```python
from build123d import *

# Parameters (mm, degrees)
F0_W     = 1500
F0_H     = 1000
F1_DEPTH = 1500
F2_W     = 300
F2_H     = 80
F3_DEPTH = 1000
F4_W     = 290.798738
F4_H     = 1259.663105
F4_W_2   = 753.015757
F5_DEPTH = 25
F6_W     = 1170.94978
F6_H     = 737.592996
F7_DEPTH = 25
F8_W     = 501.033828
F8_H     = 1276.894093
F9_DEPTH = 25


with BuildPart() as f1:
    # F0 (on Front) → F1 (new body)
    with BuildSketch(Plane.XZ):
        with Locations((750, 500)):
            Rectangle(F0_W, F0_H)
    extrude(amount=F1_DEPTH)

    # F2 (on face) → F3 (cut)
    with BuildSketch(Plane.XY.offset(1000)):
        with Locations((250, -1460)):
            Rectangle(F2_W, F2_H)
        with Locations((1250, -1460)):
            Rectangle(F2_W, F2_H)
    extrude(amount=-F3_DEPTH, mode=Mode.SUBTRACT)

    # F4 (on face) → F5 (cut)
    with BuildSketch(Plane.XY.offset(1000)):
        with Locations((286.252491, -629.831552)):
            Rectangle(F4_W, F4_H)
        with Locations((988.761067, -629.831552)):
            Rectangle(F4_W_2, F4_H)
    extrude(amount=-F5_DEPTH, mode=Mode.SUBTRACT)

    # F6 (on face) → F7 (cut)
    with BuildSketch(Plane(origin=(0, 0, 0), x_dir=(0, -1, 0), z_dir=(-1, 0, 0))):
        with Locations((685.361821, 483.926624)):
            Rectangle(F6_W, F6_H)
    extrude(amount=-F7_DEPTH, mode=Mode.SUBTRACT)

    # F8 (on face) → F9 (cut)
    with BuildSketch(Plane(origin=(0, 0, 0), x_dir=(1, 0, 0), z_dir=(0, 0, -1))):
        with Locations((446.271874, 638.447046)):
            Rectangle(F8_W, F8_H)
    extrude(amount=-F9_DEPTH, mode=Mode.SUBTRACT)


solid = f1.part
```
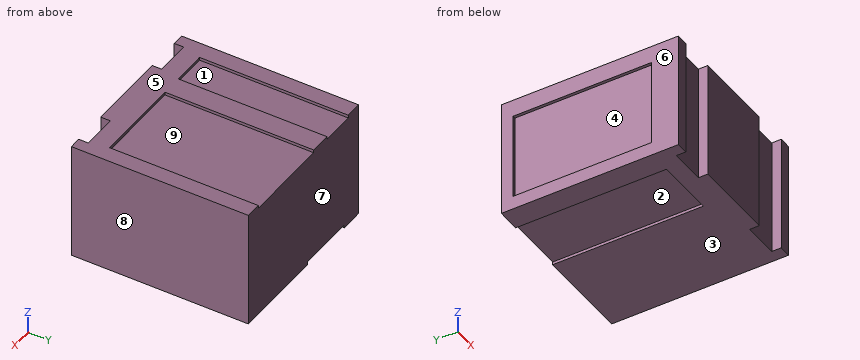
Design review of the part built by this model. Coordinates are the model's own, in mm. Face numbers are marked on the shaded views. A direction names the side the tool comes from. Round coordinates to 2 decimals unless told otherwise and drop trailing zeros. Write each loop counter-clockwise with the first axis right and the second up, starting at its lowest first coordinate (ties: lowest second). Pieces come first, ordered by that corner, then holes.
Item 1: We need section B-B on x = 348. Write out the cut boundary in (y, z).
Item 2: Clearance check with flat-ended pins moving along their axes: pin 1 Ø10 at (x, y) = (469.5, -856) entering from -Z; pin 2 Ø5 at (y, z) = (-514.5, 172) entering from -X; pin 3 Ø1.5 at (x, z) = (1220, 791.5) entering from -Y. State where each tip first meets the part, or that it passes through.
Item 3: We need section D-D on z = 932. Write out the cut boundary in (x, y).
Item 4: We need section C-C on y = -757. Write out the cut boundary in (x, z).
Item 5: The part is to be moulded in two halves that separate along X. For the marked faces 6, 7, 8 and 9, say which applies: +X half, -X half, draft (parallel to the pull), parting line (faces both ways), or undercut.
Item 6: For probe 1 along X at (y, z) = (-575, 244.5); probe 2 along Z at (x, y) = (1089, -923); probe 3 along Y at (x, z) = (219, 958.5), list the stretches that pass through material, from the lowest coordinate up.
Item 7: We need section A-A on z = 773. Write out the cut boundary in (x, y).
Item 8: For the marked faces 1, 2, 3, 4 and 5, list the 3-axis set-ups (+Z, -Z, +X, -X, +Y, -Y) from which the entire face can be reached by the end or side of a thin tool; tool diameter is ignored.
Returned:
1. outline: (-1420, 0) - (-1276.89, 0) - (-1276.89, 25) - (0, 25) - (0, 975) - (-1259.66, 975) - (-1259.66, 1000) - (-1420, 1000) - close
2. pin 1: stops at z = 25
2. pin 2: stops at x = 25
2. pin 3: stops at y = -1420
3. outline: (0, -1500) - (100, -1500) - (100, -1420) - (400, -1420) - (400, -1500) - (1100, -1500) - (1100, -1420) - (1400, -1420) - (1400, -1500) - (1500, -1500) - (1500, 0) - (0, 0) - close
4. outline: (0, 0) - (195.75, 0) - (195.75, 25) - (696.79, 25) - (696.79, 0) - (1500, 0) - (1500, 1000) - (1365.27, 1000) - (1365.27, 975) - (612.25, 975) - (612.25, 1000) - (431.65, 1000) - (431.65, 975) - (140.85, 975) - (140.85, 1000) - (0, 1000) - (0, 852.72) - (25, 852.72) - (25, 115.13) - (0, 115.13) - close
5. face 6: -X half
5. face 7: draft
5. face 8: +X half
5. face 9: undercut
6. probe 1: x = 25 to 1500
6. probe 2: z = 0 to 975
6. probe 3: y = -1420 to 0
7. outline: (0, -1500) - (100, -1500) - (100, -1420) - (400, -1420) - (400, -1500) - (1100, -1500) - (1100, -1420) - (1400, -1420) - (1400, -1500) - (1500, -1500) - (1500, 0) - (0, 0) - (0, -99.89) - (25, -99.89) - (25, -1270.84) - (0, -1270.84) - close
8. face 1: +Z, +Y
8. face 2: -Z, +Y
8. face 3: -Z, +X, -X, +Y, -Y
8. face 4: -X
8. face 5: +Z, +X, -X, +Y, -Y
